Could you check a few things on this model? Use its own coordinates, in mm. Face numbers are marked on the shaded views. A direction names the side the tool comes from. Coordinates: 2 decimals unless noted, no trailing zeros. Loops run counter-clockwise (first coordinate to the right, second up) from the corner with the lowest first, then second, coordinate; pieces in that order, holes last.
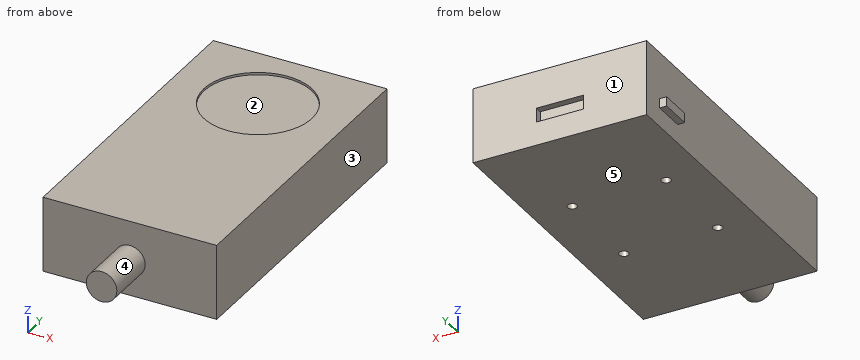
Autodesk Fusion 360 part; units mm, degrees
sketch "Sketch1" plane through (0, 0, 0) normal (0, 0, 1) x (1, 0, 0)
  line L0 (-18.5, 33) -> (18.5, 33)
  line L1 (18.5, 33) -> (18.5, -33)
  line L2 (18.5, -33) -> (-18.5, -33)
  line L3 (-18.5, -33) -> (-18.5, 33)
  line L4 (-18.5, 33) -> (18.5, -33) construction
  line L5 (18.5, 33) -> (-18.5, -33) construction
  dimension "d1" = 37
  dimension "d2" = 66
extrude "Extrude1" add sketch "Sketch1" along normal blind 16 makes body 1
sketch "Sketch2" plane through (0, 0, 0) normal (0, 0, 1) x (1, 0, 0)
  line L0 (10, -10) -> (-10, -10) construction
  line L1 (-10, -10) -> (-10, 10) construction
  line L2 (-10, 10) -> (10, 10) construction
  line L3 (10, 10) -> (10, -10) construction
  line L4 (10, -10) -> (-10, 10) construction
  line L5 (-10, -10) -> (10, 10) construction
  circle A0 centre (10, 10) radius 1
  circle A1 centre (10, -10) radius 1
  circle A2 centre (-10, 10) radius 1
  circle A3 centre (-10, -10) radius 1
  dimension "d5" = 2
  dimension "d6" = 2
  dimension "d7" = 2
  dimension "d8" = 2
extrude "Extrude2" cut sketch "Sketch2" along normal blind 2.5 bodies 1
sketch "Sketch3" plane through (0, -33, 0) normal (0, -1, 0) x (1, 0, 0)
  line L0 (-18.5, 0) -> (18.5, 0)
  line L1 (18.5, 0) -> (18.5, 16)
  line L2 (18.5, 16) -> (-18.5, 16)
  line L3 (-18.5, 16) -> (-18.5, 0)
  circle A0 centre (0, 7.5245) radius 3.25
  dimension "d11" = 6.5
sketch "Sketch4" plane through (0, -33, 0) normal (0, -1, 0) x (1, 0, 0)
  line L0 (-18.5, 0) -> (18.5, 0)
  line L1 (18.5, 0) -> (18.5, 16)
  line L2 (18.5, 16) -> (-18.5, 16)
  line L3 (-18.5, 16) -> (-18.5, 0)
  circle A0 centre (0.0221, 7.5311) radius 3.25
  dimension "d12" = 6.5
extrude "Extrude3" add sketch "Sketch4" along normal blind 11 contours A0 bodies 1
sketch "Sketch5" plane through (0, 0, 16) normal (0, 0, 1) x (-1, 0, 0)
  line L0 (18.5, 33) -> (-18.5, 33)
  line L1 (-18.5, 33) -> (-18.5, -33)
  line L2 (-18.5, -33) -> (18.5, -33)
  line L3 (18.5, -33) -> (18.5, 33)
  circle A0 centre (0, -16.6341) radius 11.5
  dimension "d15" = 23
extrude "Extrude4" cut sketch "Sketch5" against normal blind 0.5 contours A0 bodies 1
sketch "Sketch6" plane through (-18.5, 0, 0) normal (-1, 0, 0) x (0, -1, 0)
  line L0 (-33, 0) -> (33, 0)
  line L1 (33, 0) -> (33, 16)
  line L2 (33, 16) -> (-33, 16)
  line L3 (-33, 16) -> (-33, 0)
  line L4 (-28, 6) -> (-21, 6)
  line L5 (-21, 6) -> (-21, 4)
  line L6 (-21, 4) -> (-28, 4)
  line L7 (-28, 4) -> (-28, 6)
extrude "Extrude5" add sketch "Sketch6" along normal blind 1.5 separate body contours L4 L5 L6 L7 makes body 2
sketch "Sketch7" plane through (0, 33, 0) normal (0, 1, 0) x (-1, 0, 0)
  line L0 (-18.5, 0) -> (18.5, 0)
  line L1 (18.5, 0) -> (18.5, 16)
  line L2 (18.5, 16) -> (-18.5, 16)
  line L3 (-18.5, 16) -> (-18.5, 0)
  line L4 (-5, 8) -> (5, 8)
  line L5 (5, 8) -> (5, 5)
  line L6 (5, 5) -> (-5, 5)
  line L7 (-5, 5) -> (-5, 8)
extrude "Extrude6" cut sketch "Sketch7" against normal blind 1.5 contours L4 L5 L6 L7 bodies 1
combine "Combine1" operation add target body 1 tool bodies 2
1) We'd pull the mould along Y, two halves only. Please class the marked faces 1, 2 and 3: released by +Y, released by -Y, zero draft, split by the parting line, or undercut.
2) Imagine slicing it at D-D on y = -30.5. List the corners of the cut face in (x, z) for me, plus the area to 3 significant figures.
3) Will these pins go through, and if not, where does the flat tip stop? pin 1 (0.8 mm diameter, centred on x = -19.5, z = 5, fed in from -Y); pin 2 (5 mm diameter, centred on x = 6.5, z = 11, fed in from -Y); pin 3 (1 mm diameter, centred on x = 10, y = 10, fed in from -Z).
4) Imagine slicing it at B-B on x = 0. List the corners of the cut face in (y, z) for me.
5) Imagine slicing it at C-C on z = 3.25. List the corners of the cut face in (x, y) for me, plus the area to 3 significant figures.
6) For the marked faces 4 and 5, which set-ups out of +Z, -Z, +X, -X, +Y, -Y let a thin tool reach every point of the face, with its end or its side?
7) Imagine slicing it at A-A on y = -10. List the corners of the cut face in (x, z) for me, plus the area to 3 significant figures.
8) If I drill on L1, parallel to Y at x = 10, z = 1; L2, parallel to Y at x = 0, z = 15.7; L3, parallel to Z at x = -7, y = 17.5, over which ranges is the centre line in solid material (lowest first)?
Solved:
1. face 1: released by +Y
1. face 2: undercut
1. face 3: zero draft
2. outline: (-18.5, 0) - (18.5, 0) - (18.5, 16) - (-18.5, 16) - close
2. area: 592 mm2
3. pin 1: stops at y = 21
3. pin 2: stops at y = -33
3. pin 3: stops at z = 2.5
4. outline: (-44, 4.28) - (-33, 4.28) - (-33, 0) - (33, 0) - (33, 5) - (31.5, 5) - (31.5, 8) - (33, 8) - (33, 16) - (28.13, 16) - (28.13, 15.5) - (5.13, 15.5) - (5.13, 16) - (-33, 16) - (-33, 10.78) - (-44, 10.78) - close
5. outline: (-18.5, -33) - (18.5, -33) - (18.5, 33) - (-18.5, 33) - close
5. area: 2,440 mm2
6. face 4: -Y
6. face 5: -Z, +X, -X, +Y, -Y
7. outline: (-18.5, 0) - (-11, 0) - (-11, 2.5) - (-9, 2.5) - (-9, 0) - (9, 0) - (9, 2.5) - (11, 2.5) - (11, 0) - (18.5, 0) - (18.5, 16) - (-18.5, 16) - close
7. area: 582 mm2
8. L1: y = -33 to -11, -9 to 9, 11 to 33
8. L2: y = -33 to 5.13, 28.13 to 33
8. L3: z = 0 to 15.5
